```python
from build123d import *

# Parameters (mm, degrees)
CYLINDER_R     = 0.25
CYLINDER_DEPTH = 2.5
PAD_DEPTH      = 0.35
PAD001_DEPTH   = 0.5
PRISM_DEPTH    = 0.35
PAD002_DEPTH   = 0.45
POCKET_DEPTH   = 0.45


with BuildPart() as part:
    # Cylinder → Cylinder (join)
    with BuildSketch(Plane.XY):
        Circle(CYLINDER_R)
    extrude(amount=CYLINDER_DEPTH)

    # Cone → Cone (revolve)
    with BuildSketch(Plane(origin=(0, 0, 2), x_dir=(1, 0, 0), z_dir=(0, 0, -1))):
        Polygon((0, 0), (0.15, 0), (0.3, 2), (0, 2), align=None)
    cone = revolve(axis=Axis((0, 0, 2), (0, -1, 0)))

    # Mirrored: Cone across XZ
    add(cone.mirror(Plane.XZ))

    # Sketch (on Face1 of Mirrored) → Pad (join)
    with BuildSketch(Plane(origin=(0, 0, 0), x_dir=(1, 0, 0), z_dir=(0, 0, -1))):
        Polygon((0.779423, -0.45), (0.779423, 0.45), (0, 0.9), (-0.779423, 0.45), (-0.779423, -0.45), (0, -0.9), align=None)
    extrude(amount=-PAD_DEPTH)

    # Sphere → Sphere (revolve)
    with BuildSketch(Plane(origin=(0, 0, -0.75), x_dir=(1, 0, 0), z_dir=(0, -1, 0))):
        with BuildLine():
            ThreePointArc((0, -1), (1, 0), (0, 1))
            Line((0, 1), (0, -1))
        make_face()
    revolve(axis=Axis((0, 0, -0.75), (0, 0, 1)))

    # Sketch001 (on Sphere) → Pad001 (join, symmetric)
    with BuildSketch(Plane(origin=(0, 0, -0.75), x_dir=(1, 0, 0), z_dir=(0, -1, 0))):
        with BuildLine():
            Line((-3, 0.55), (1.8, 0.55))
            ThreePointArc((2.9, -0.55), (2.577817, 0.227817), (1.8, 0.55))
            Line((2.9, -0.55), (2.9, -0.8))
            Line((2.9, -0.8), (1.9, -0.8))
            Line((1.9, -0.8), (1.9, -0.55))
            Line((1.9, -0.55), (-3, -0.55))
            Line((-3, -0.55), (-3, 0.55))
        make_face()
    extrude(amount=PAD001_DEPTH, both=True)

    # Prism → Prism (join)
    with BuildSketch(Plane(origin=(-1.5, 0, -0.75), x_dir=(0, -0.866025, 0.5), z_dir=(-1, 0, 0))):
        Polygon((0.9, 0), (0.45, 0.779423), (-0.45, 0.779423), (-0.9, 0), (-0.45, -0.779423), (0.45, -0.779423), align=None)
    extrude(amount=PRISM_DEPTH)

    # Sketch002 (on Sphere) → Pad002 (join, symmetric)
    with BuildSketch(Plane(origin=(0, 0, -0.75), x_dir=(1, 0, 0), z_dir=(0, -1, 0))):
        with BuildLine():
            Line((-3, -0.5), (-3, 0.5))
            Line((-3, 0.5), (1.754555, 0.5))
            ThreePointArc((2.85, -0.5), (2.496175, 0.212404), (1.754555, 0.5))
            Line((2.85, -0.5), (2.85, -0.8))
            Line((2.85, -0.8), (1.95, -0.8))
            Line((1.95, -0.8), (1.95, -0.5))
            Line((1.95, -0.5), (-3, -0.5))
        make_face()
    extrude(amount=PAD002_DEPTH, both=True)

    # Sketch002 (on Sphere) → Pocket (cut, symmetric)
    with BuildSketch(Plane(origin=(0, 0, -0.75), x_dir=(1, 0, 0), z_dir=(0, -1, 0))):
        with BuildLine():
            Line((-3, -0.5), (-3, 0.5))
            Line((-3, 0.5), (1.754555, 0.5))
            ThreePointArc((2.85, -0.5), (2.496175, 0.212404), (1.754555, 0.5))
            Line((2.85, -0.5), (2.85, -0.8))
            Line((2.85, -0.8), (1.95, -0.8))
            Line((1.95, -0.8), (1.95, -0.5))
            Line((1.95, -0.5), (-3, -0.5))
        make_face()
    extrude(amount=POCKET_DEPTH, both=True, mode=Mode.SUBTRACT)


solid = part.part
```
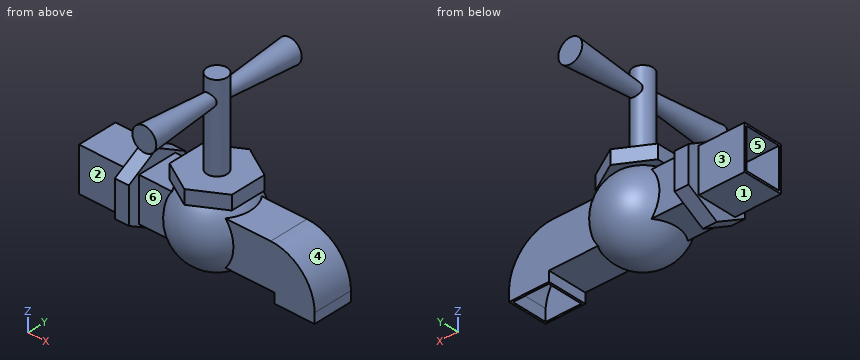
Input: part model. Units: mm. Frame: model coordinates. Face numbers are marked on the shaded views. A direction names the side the tool comes from. Coordinates: 2 decimals unless noted, no trailing zeros. Order: outer loops, then holes, each group sorted by start corner. A loop starts at its lowest first (then second) coordinate and runs counter-clockwise, first axis right, second up. Notation, with made-up numbers: (-24.75, 23) - (6.25, 23) arc R17 cw to (6.25, 34) - close; hole circle Ø11 at (76.5, -7). An arc over 180 degrees is marked (long way). Put each result on its own line as item: value.
1. Cut plane D-D on z = 2. Return the cut outline in (x, y), then the cut area to 3 significant figures.
Report:
outline: (-0.3, -2) - (0.3, -2) - (0.16, -0.19) arc R0.25 ccw to (0.16, 0.19) - (0.3, 2) - (-0.3, 2) - (-0.16, 0.19) arc R0.25 ccw to (-0.16, -0.19) - close
area: 1.85 mm2
2. Reachability of the marked faces 1, 2 and 3 from +Z, -Z, +X, -X, +Y, -Y: full face, straight path, thin tool, end or side. Return the list, or none.
Report:
face 1: -Z, -X, +Y, -Y
face 2: +Z, -Z, -X, -Y
face 3: +Z, -Z, -X, +Y
3. Cut plane C-C on x = -0.5. Return the cut outline in (y, z).
Report:
outline: (-0.61, 0) - (-0.43, 0) arc R0.87 ccw (long way) to (0.43, 0) - (0.61, 0) - (0.61, 0.35) - (-0.61, 0.35) - close; hole (-0.45, -1.25) - (0.45, -1.25) - (0.45, -0.25) - (-0.45, -0.25) - close
4. Contact query for flat-ended pins moving along their axis: pin 1 Ø1 at (x, z) = (1.5, -0.5) entering from -Y; pin 2 Ø1.2 at (x, y) = (0.5, 0) entering from +Z; pin 3 Ø1 at (y, z) = (0.5, 1) entering from +X; pin 4 Ø1.2 at (x, z) = (-2, -1) entering from +Y. Output: stop coordinate, or through.
Report:
pin 1: stops at y = -0.5
pin 2: stops at z = 2.5
pin 3: stops at x = 0.25
pin 4: stops at y = 0.78
5. Cut plane B-B on z = -0.1. Return the cut outline in (x, y).
Report:
outline: (-1.85, -0.43) - (-1.5, -0.43) - (-1.5, 0.43) - (-1.85, 0.43) - close; circle Ø1.52 at (0, 0)
6. Line query: line 1 along Z through (x, y) = (-1.7, 0.3); line 2 along Y through (x, z) = (0.1, -0.45); line 3 along X through (y, z) = (0.55, -0.65). Output: solid intervals per line, ascending.
Report:
line 1: z = -1.48 to -1.25, -0.25 to -0.02
line 2: y = -0.95 to -0.45, 0.45 to 0.95
line 3: x = -1.85 to -1.5, -0.83 to 0.83
7. Draft query along X for the marked faces 4, 5 and 6. Return one class per face: pulls with the +X half, pulls with the -X half, needs draft (parallel to the pull), parting line crosses it, or undercut.
Report:
face 4: pulls with the +X half
face 5: needs draft
face 6: undercut
8. Cut plane A-A on x = 1.2. Return the cut outline in (y, z).
Report:
outline: (-0.5, -1.3) - (0.5, -1.3) - (0.5, -0.2) - (-0.5, -0.2) - close; hole (-0.45, -1.25) - (0.45, -1.25) - (0.45, -0.25) - (-0.45, -0.25) - close
